from build123d import *

# Parameters (mm, degrees)
F1_DEPTH = 830
F2_R     = 95
F5_DEPTH = 540.001


with BuildPart() as f1:
    # F0 (on Front) → F1 (new body)
    with BuildSketch(Plane.XZ):
        Polygon((-645.752296802, 876.8817598489), (-835.752296802, 717.4528299252), (-835.752296802, 156.8817598489), (-705.752296802, 156.8817598489), (-705.752296802, 96.8817598489), (-425.752296802, 96.8817598489), (-425.752296802, 156.8817598489), (-295.752296802, 156.8817598489), (-295.752296802, 459.7680024409), align=None)
    extrude(amount=F1_DEPTH)

    # F2 (on face) → F4 section 0
    with BuildSketch(Plane.YZ.offset(-295.752296802)):
        Polygon((-220, 459.7680024409), (-360, 459.7680024409), (-423.5085296109, 349.7680024409), (-156.4914703891, 349.7680024409), align=None)
    # F3 (on face) → F4 section 1
    with BuildSketch(Plane(origin=(-698.5892714061, 0, 832.546273946), x_dir=(0.7660444431, 0, 0.6427876097), z_dir=(-0.6427876097, 0, 0.7660444431))):
        Polygon((-41.0262282055, -733.5085296109), (68.9737717945, -670), (68.9737717945, -530), (-41.0262282055, -466.4914703891), align=None)
    loft(mode=Mode.SUBTRACT)

    # F2 (on face) → F5 (cut, through all)
    with BuildSketch(Plane.YZ.offset(-295.752296802)):
        with Locations((-610, 316.8817598489)):
            Circle(F2_R)
    extrude(amount=-F5_DEPTH, mode=Mode.SUBTRACT)


solid = f1.part
CAD build for the part. Positions are in the model's coordinates, mm. A direction names the side the tool comes from. Round coordinates to 2 decimals unless told otherwise and drop trailing zeros. One line per question, with ' | ' between items. Start each with the question number.
Item 1: Pin check, flat tips, straight feed: pin 1 Ø2 at (x, y) = (-458.5, -456.5) entering from +Z; pin 2 Ø18 at (y, z) = (-343, 119) entering from -X; pin 3 Ø1.5 at (y, z) = (-176.5, 533.5) entering from +X; pin 4 Ø10 at (x, z) = (-703.5, 382) entering from +Y. Stop position of each tip, or through.
Item 2: Two-plate mould, pull along Z, no slides. Class faces 1 (the flat face through (-507.19, -202.4, 711.75)), 2 (the flat face through (-772, -409, 156.882)), 3 (the cylindrical face through (-561.972, -519.387, 345.417)): pulls with the +Z half, pulls with the -Z half, needs draft (parallel to the pull), parting line crosses it, or undercut.
Item 3: Which spindle directions (+Z, -Z, +X, -X, +Y, -Y) get a long thin tool onto all of the face, cutting with end or side? Do faces 4 (the flat face through (-705.752, -409, 127)), 5 (the flat face through (-835.752, -409, 441)), 6 (the flat face through (-362, -409, 156.882)). Say none if no direction does.
Item 4: Wall check: line 1 (Y direction, x = -460.5, z = 316); line 2 (Y direction, x = -541, z = 746.5); line 3 (Z direction, x = -705, y = -663). Give the ranges that are in metal, low to high.
Responses:
1) pin 1: stops at z = 521.86 | pin 2: stops at x = -705.75 | pin 3: stops at x = -356.99 | pin 4: stops at y = 0
2) face 1: pulls with the +Z half | face 2: pulls with the -Z half | face 3: undercut
3) face 4: -Z, -X, +Y, -Y | face 5: +Z, -Z, -X, +Y, -Y | face 6: -Z, +X, +Y, -Y
4) line 1: y = -830 to -705, -515 to 0 | line 2: y = -830 to -577.64, -433.03 to 0 | line 3: z = 96.88 to 238.04, 395.72 to 779.88
